Geometry: final body of the model. Coordinates: model frame, mm. A direction names the side the tool comes from. Round coordinates to 2 decimals unless told otherwise and drop trailing zeros. Loops run counter-clockwise (first coordinate to the right, second up) from the corner with the lowest first, then second, coordinate; pieces in that order, holes last. Notation, with made-up numbers: (62, -15) - (89, -15) arc R8 ccw to (89, -3) - close; hole circle Ø3 at (16.5, 71.5). An arc over 180 degrees is marked (long way). Use CSV: the item, a comma, the result in double quotes.
from build123d import *

# Parameters (mm, degrees)
F1_DEPTH = 3
F2_R     = 1.49999


# Not quite as in the source:
# - a fillet or chamfer is up to 0.001 mm smaller than in the source, because OpenCascade refuses the exact size


with BuildPart() as f1:
    # F0 (on Top) → F1 (new body)
    with BuildSketch(Plane.XY):
        with BuildLine():
            ThreePointArc((0, -6.5), (-6.5, 0), (0, 6.5))
            Line((0, 6.5), (22, 6.5))
            ThreePointArc((22, 6.5), (28.5, 0), (22, -6.5))
            Line((22, -6.5), (22, -9.5))
            ThreePointArc((22, -9.5), (31.5, 0), (22, 9.5))
            Line((22, 9.5), (0, 9.5))
            ThreePointArc((0, 9.5), (-9.5, 0), (0, -9.5))
            Line((0, -9.5), (20, -9.5))
            Line((20, -9.5), (20, -6.5))
            Line((20, -6.5), (0, -6.5))
        make_face()
    extrude(amount=F1_DEPTH)

    # F2 (radius 1.5 in the source; OpenCascade refuses exactly that, so slightly less here)
    f2_edges = [f1.edges().sort_by_distance(p)[0] for p in [
        (20, -9.5, 1.5),
        (20, -6.5, 1.5),
        (22, -6.5, 1.5),
        (22, -9.5, 1.5),
    ]]
    fillet(f2_edges, radius=F2_R)


solid = f1.part
Item 1: Material intervals for line 1 (Y direction, x = 13, z = 2.45); line 2 (X direction, y = 0, z = 0.5); line 3 (Y direction, x = -5, z = 1.5), sorted ascending.
Final values:
line 1,"y = -9.5 to -6.5, 6.5 to 9.5"
line 2,"x = -9.5 to -6.5, 28.5 to 31.5"
line 3,"y = -8.08 to -4.15, 4.15 to 8.08"
Item 2: Pin query (flat end, axial travel): P1, Ø1.5, axis at x = 4.5, y = -7.5, coming from the -Z side. Return the tip coordinate at first contact, or that it passes through.
Final values:
P1,"stops at z = 0"
Item 3: Section B-B on x = 17. Return the cut outline in (y, z).
Final values:
outline,"(-9.5, 0) - (-6.5, 0) - (-6.5, 3) - (-9.5, 3) - close; (6.5, 0) - (9.5, 0) - (9.5, 3) - (6.5, 3) - close"
Item 4: Mould query, pull axis X, two halves, no side actions, for faces 1 (the cylindrical face through (22.53, -9, 1.52)), 2 (the flat face through (11, 9.5, 1)), 3 (the cylindrical face through (-9.498, 0.209, 1.479)). Classes: released by +X, released by -X, zero draft, split by the parting line, or undercut.
Final values:
face 1,"undercut"
face 2,"zero draft"
face 3,"released by -X"
Item 5: Reachability of faces 4 (the cylindrical face through (-6.5, -0.1, 1.5)), 5 (the cylindrical face through (19.55, -9.07, 1.52)), 6 (the flat face through (9, -9.5, 1)) from +Z, -Z, +X, -X, +Y, -Y: full face, straight path, thin tool, end or side. Return the list, or none.
Final values:
face 4,"+Z, -Z"
face 5,"+Z, -Z, -Y"
face 6,"+Z, -Z, +X, -X, -Y"
Item 6: Section A-A on y = 0. Return the cut outline in (x, z), plus the area to 3 significant figures.
Final values:
outline,"(-9.5, 0) - (-6.5, 0) - (-6.5, 3) - (-9.5, 3) - close; (28.5, 0) - (31.5, 0) - (31.5, 3) - (28.5, 3) - close"
area,"18.0 mm²"
